```python
from build123d import *

# Parameters (mm, degrees)
SKETCH1_W           = 38
SKETCH1_H           = 53
SKETCH1_W_2         = 22
SKETCH1_H_2         = 42
BOSS_EXTRUDE1_DEPTH = 20
SKETCH4_R           = 1.5
CUT_EXTRUDE3_DEPTH  = 39.252450902
FILLET1_R           = 5
SKETCH5_R           = 1.75
CUT_EXTRUDE4_DEPTH  = 45.746508244
SKETCH5_3_R         = 2.85
SKETCH5_3_R_2       = 1.75
CUT_EXTRUDE5_DEPTH  = 3.5


with BuildPart() as part:
    # Sketch1 → Boss-Extrude1 (new body)
    with BuildSketch(Plane.XY):
        Rectangle(SKETCH1_W, SKETCH1_H)
        Rectangle(SKETCH1_W_2, SKETCH1_H_2, mode=Mode.SUBTRACT)
    extrude(amount=BOSS_EXTRUDE1_DEPTH)

    # Sketch4 → Cut-Extrude3 (cut, through all)
    with BuildSketch(Plane(origin=(0, 0, 0), x_dir=(-1, 0, 0), z_dir=(0, 0, -1))):
        with Locations((-5.1, -23.9)):
            Circle(SKETCH4_R)
        with Locations((5.1, -23.9)):
            Circle(SKETCH4_R)
        with Locations((-5.1, 23.9)):
            Circle(SKETCH4_R)
        with Locations((5.1, 23.9)):
            Circle(SKETCH4_R)
    extrude(amount=-CUT_EXTRUDE3_DEPTH, mode=Mode.SUBTRACT)

    # Fillet1
    fillet1_edges = [part.edges().sort_by_distance(p)[0] for p in [
        (19, -26.5, 10),
        (-19, -26.5, 10),
        (-19, 26.5, 10),
        (19, 26.5, 10),
    ]]
    fillet(fillet1_edges, radius=FILLET1_R)

    # Sketch5 → Cut-Extrude4 (cut, through all)
    with BuildSketch(Plane(origin=(-11, 0, 0), x_dir=(0, 0, -1), z_dir=(1, 0, 0))):
        with Locations((-14, -9)):
            Circle(SKETCH5_R)
        with Locations((-6, -9)):
            Circle(SKETCH5_R)
    extrude(amount=-CUT_EXTRUDE4_DEPTH, mode=Mode.SUBTRACT)

    # Sketch5<3> → Cut-Extrude5 (cut)
    # profile 1 of 2: a face of its own
    with BuildSketch(Plane(origin=(-11, 0, 0), x_dir=(0, 0, -1), z_dir=(1, 0, 0))):
        with Locations((-14, -9)):
            Circle(SKETCH5_3_R)
        with Locations((-14, -9)):
            Circle(SKETCH5_3_R_2, mode=Mode.SUBTRACT)
    # profile 2 of 2: a face of its own
    with BuildSketch(Plane(origin=(-11, 0, 0), x_dir=(0, 0, -1), z_dir=(1, 0, 0))):
        with Locations((-6, -9)):
            Circle(SKETCH5_3_R)
        with Locations((-6, -9)):
            Circle(SKETCH5_3_R_2, mode=Mode.SUBTRACT)
    extrude(amount=-CUT_EXTRUDE5_DEPTH, mode=Mode.SUBTRACT)


solid = part.part
```
The model under review builds one solid part; all positions refer to its coordinate system, in mm. A direction names the side the tool comes from. Give positions to 0.01 mm unless a question says otherwise; leave off trailing zeros. Write each loop counter-clockwise with the first axis right and the second up, starting at its lowest first coordinate (ties: lowest second). Pieces come first, ordered by that corner, then holes.
(1) Consider section A-A, the plane y = -0.5. Give the boundary of the cut face in (x, z).
(2) For P1, Ø2, axis at y = -9, z = 14, coming from the -X side; P2, Ø2.5, axis at x = 5.1, y = -23.9, coming from the +Z side, all flat-tipped, find the tip position at first contact; note any pin that passes through.
(3) Tool access review of faces 1 (the cylindrical face through (-16.718, -7.265, 6.228)), 2 (the flat face through (0, 21, 10)), 3 (the cylindrical face through (-12.726, -7.074, 16.101)), 4 (the cylindrical face through (17.5, -25.07, 10.14)): name each direction out of +Z, -Z, +X, -X, +Y, -Y from which nothing blocks a thin tool from reaching the whole face with its end or side.
(4) Consider section D-D, the plane y = -9. Give the boundary of the cut face in (x, z), and give its area (3 significant figures).
(5) To check wall thickness, follow L1, parallel to Y at x = 5, z = 2.5; L2, parallel to X at y = -8, z = 2.25; L3, parallel to Y at x = 8, z = 8.25. State the ranges of each line that lie inside material, in increasing order.
(6) Consider section B-B, the plane z = 2.5. Give the boundary of the cut face in (x, y), and give its area (3 significant figures).
(7) Consider section C-C, the plane x = -5.1. Give the boundary of the cut face in (y, z).
(8) The part is to be moulded in two halves that separate along X. For faces 5 (the flat face through (19, 0, 10)), 6 (the flat face through (-14.5, -11, 14)), 7 (the flat face through (0, 26.5, 10)), say which applies: released by +X, released by -X, zero draft, split by the parting line, or undercut.
Returned:
1. outline: (-19, 0) - (-11, 0) - (-11, 20) - (-19, 20) - close; (11, 0) - (19, 0) - (19, 20) - (11, 20) - close
2. P1: stops at x = 11
2. P2: passes through
3. face 1: -X
3. face 2: +Z, -Z
3. face 3: none
3. face 4: +Z, -Z, +X, -Y
4. outline: (-19, 0) - (-11, 0) - (-11, 3.15) - (-14.5, 3.15) - (-14.5, 4.25) - (-19, 4.25) - close; (-19, 7.75) - (-14.5, 7.75) - (-14.5, 8.85) - (-11, 8.85) - (-11, 11.15) - (-14.5, 11.15) - (-14.5, 12.25) - (-19, 12.25) - close; (-19, 15.75) - (-14.5, 15.75) - (-14.5, 16.85) - (-11, 16.85) - (-11, 20) - (-19, 20) - close; (11, 0) - (19, 0) - (19, 20) - (11, 20) - close
4. area: 249 mm2
5. L1: y = -26.5 to -25.4, -22.4 to -21, 21 to 22.4, 25.4 to 26.5
5. L2: x = -19 to -11, 11 to 19
5. L3: y = -26.5 to -21, 21 to 26.5
6. outline: (-19, -21.5) arc R5 ccw to (-14, -26.5) - (14, -26.5) arc R5 ccw to (19, -21.5) - (19, 21.5) arc R5 ccw to (14, 26.5) - (-14, 26.5) arc R5 ccw to (-19, 21.5) - close; hole (-11, -21) - (11, -21) - (11, 21) - (-11, 21) - close; hole circle Ø3 at (-5.1, -23.9); hole circle Ø3 at (-5.1, 23.9); hole circle Ø3 at (5.1, -23.9); hole circle Ø3 at (5.1, 23.9)
6. area: 1,040 mm2
7. outline: (-26.5, 0) - (-25.4, 0) - (-25.4, 20) - (-26.5, 20) - close; (-22.4, 0) - (-21, 0) - (-21, 20) - (-22.4, 20) - close; (21, 0) - (22.4, 0) - (22.4, 20) - (21, 20) - close; (25.4, 0) - (26.5, 0) - (26.5, 20) - (25.4, 20) - close
8. face 5: released by +X
8. face 6: undercut
8. face 7: zero draft
